```python
from build123d import *

# Parameters (mm, degrees)
SKETCH4_R                     = 3.25
SKETCH4_R_2                   = 1.5
BOSS_EXTRUDE1_DEPTH           = 14.5
BOSS_EXTRUDE1_TAPER           = 1
BOSS_EXTRUDE1_OTHER_WAY_DEPTH = 1
SKETCH5_R                     = 2
CUT_EXTRUDE1_DEPTH            = 14.5


with BuildPart() as part:
    # Sketch3 → Revolve1 (revolve)
    with BuildSketch(Plane(origin=(0, 0, 0), x_dir=(0, 0, -1), z_dir=(1, 0, 0))):
        with BuildLine():
            Line((-5.5, 13), (0.74, 13))
            ThreePointArc((0.74, 13), (1.672291774, 8.668530015), (2, 4.25))
            Line((2, 4.25), (0, 4.25))
            Line((0, 4.25), (0, 3.25))
            Line((0, 3.25), (5.5, 3.25))
            Line((5.5, 3.25), (5.5, 4.25))
            Line((5.5, 4.25), (3, 4.25))
            ThreePointArc((3, 4.25), (2.672291774, 8.668530015), (1.74, 13))
            Line((1.74, 13), (5.5, 13))
            Line((5.5, 13), (5.5, 14))
            Line((5.5, 14), (3, 14))
            Line((3, 14), (3, 15.5))
            Line((3, 15.5), (-3, 15.5))
            Line((-3, 15.5), (-3, 14))
            Line((-3, 14), (-5.5, 14))
            Line((-5.5, 14), (-5.5, 13))
        make_face()
    revolve(axis=Axis((0, 0, 77.747530796), (0, 0, -1)))

    # Sketch4 → Boss-Extrude1 (add)
    with BuildSketch(Plane.XY):
        Circle(SKETCH4_R)
        Circle(SKETCH4_R_2, mode=Mode.SUBTRACT)
    extrude(amount=BOSS_EXTRUDE1_DEPTH, taper=BOSS_EXTRUDE1_TAPER)

    # Sketch4 → Boss-Extrude1 other way (add)
    with BuildSketch(Plane.XY):
        Circle(SKETCH4_R)
        Circle(SKETCH4_R_2, mode=Mode.SUBTRACT)
    extrude(amount=-BOSS_EXTRUDE1_OTHER_WAY_DEPTH)

    # Sketch5 → Cut-Extrude1 (cut)
    with BuildSketch(Plane(origin=(0, 0, -5.5), x_dir=(-1, 0, 0), z_dir=(0, 0, -1))):
        with Locations((0, 7.75)):
            Circle(SKETCH5_R)
        with Locations((6.711696879, -3.875)):
            Circle(SKETCH5_R)
        with Locations((-6.711696879, -3.875)):
            Circle(SKETCH5_R)
    extrude(amount=-CUT_EXTRUDE1_DEPTH, mode=Mode.SUBTRACT)


solid = part.part
```
CAD build for the part. Positions are in the model's coordinates, mm. A direction names the side the tool comes from. Round coordinates to 2 decimals unless told otherwise and drop trailing zeros. Write each loop counter-clockwise with the first axis right and the second up, starting at its lowest first coordinate (ties: lowest second). Pieces come first, ordered by that corner, then holes. Notation, with made-up numbers: M 88.5,16.5 L 128.5,16.5 A20 ccw 128.5,51.5 Z; hole C -2.75,49.5 d9. An arc over 180 degrees is marked long. One line per question, with ' | ' between items.
1. Probe L1, parallel to X at y = 0, z = -4.4; L2, parallel to Z at x = 8, y = 9; L3, parallel to Z at x = 13.5, y = 0. List the from-to ranges inside material, lowest first. Write a range as from..to.
Working result:
L1: -14..-13, -4.25..-3.25, 3.25..4.25, 13..14 | L2: -2..-1 | L3: -5.5..5.5
2. Cut at C-C on z = 10.5. Write the cut outline in (x, y).
Working result:
outline: C 0,0 d6.13; hole C 0,0 d3.37
3. Cut at D-D on z = 7.5. Write the cut outline in (x, y).
Working result:
outline: C 0,0 d6.24; hole C 0,0 d3.26
4. Which spindle directions (+Z, -Z, +X, -X, +Y, -Y) get a long thin tool onto all of the face, cutting with end or side? Do faces 1 (the cylindrical face through (3.584, 2.285, -0.986)), 2 (the cylindrical face through (15.368, -2.018, 0.042)), 3 (the cylindrical face through (3.584, 2.285, -4.232)). Say none if no direction does.
Working result:
face 1: +Z | face 2: +Z, -Z | face 3: -Z
5. Cut at B-B on x = -0.5. Count the separate pieces of the cut face and the enclosed holes in it, and give its area (3 significant figures).
Working result:
separate pieces: 3 | enclosed holes: 0 | area: 113 mm2
6. Mould opens along X. For faces 4 (the conical face through (1.553, -0.489, 7.352)), 5 (the cylindrical face through (2, 7.8, -2.2)), 6 (the cylindrical face through (-5.362, 12.932, 4.268)), 7 (the flat face through (-8, -12, 3)) say: pulls with the +X half, pulls with the -X half, needs draft (parallel to the pull), parting line crosses it, or undercut.
Working result:
face 4: undercut | face 5: undercut | face 6: parting line crosses it | face 7: needs draft
7. Pin check, flat tips, straight feed: pin 1 Ø6 at (x, z) = (12, 3) entering from +Y; pin 2 Ø5 at (x, z) = (-6.5, 2) entering from -Y (3 decimals); pin 3 Ø4.5 at (x, y) = (0, 7.75) entering from -Z. Stop position of each tip, or through.
Working result:
pin 1: y = 12.62 | pin 2: y = -14.975 | pin 3: z = -2.97
8. Cut at A-A on z = 1.25. Write the cut outline in (x, y).
Working result:
outline: C 0,0 d31; C 0,0 d6.46; hole C 0,0 d26; hole C 0,0 d3.04
